```python
from build123d import *

# Parameters (mm, degrees)
SKETCH1_R               = 2.5
BOSS_EXTRUDE1_DEPTH     = 5
SKETCH2_R               = 2.51348819
BOSS_EXTRUDE2_DEPTH     = 1
BOSS_EXTRUDE3_DEPTH     = 3
CUT_EXTRUDE1_DEPTH      = 28.128538457
CUT_EXTRUDE1_DEPTH_BACK = 28.128538457
SKETCH5_R               = 0.5
CUT_EXTRUDE2_START      = -10
SKETCH6_R               = 1.5
CUT_EXTRUDE2_DEPTH      = 10


with BuildPart() as part:
    # Sketch1 → Boss-Extrude1 (new body)
    with BuildSketch(Plane(origin=(0, 0, -3.289858219), x_dir=(-1, 0, 0), z_dir=(0, 0, -1))):
        with BuildLine():
            Line((2.125597577, 8.274515134), (2.125597577, 18.874515134))
            ThreePointArc((2.125597577, 18.874515134), (5.125597577, 21.874515134), (8.125597577, 18.874515134))
            Line((8.125597577, 18.874515134), (8.125597577, 8.274515134))
            ThreePointArc((8.125597577, 8.274515134), (5.125597577, 5.274515134), (2.125597577, 8.274515134))
        make_face()
        with Locations((5.125597577, 18.874515134)):
            Circle(SKETCH1_R, mode=Mode.SUBTRACT)
        with Locations((5.125597577, 8.274515134)):
            Circle(SKETCH1_R, mode=Mode.SUBTRACT)
    extrude(amount=BOSS_EXTRUDE1_DEPTH)

    # Sketch2 → Boss-Extrude2 (add)
    with BuildSketch(Plane(origin=(0, 0, -3.289858219), x_dir=(-1, 0, 0), z_dir=(0, 0, -1))):
        with Locations((5.139085766, 8.274515134)):
            Circle(SKETCH2_R)
        with Locations((5.139085766, 18.874515134)):
            Circle(SKETCH2_R)
    extrude(amount=BOSS_EXTRUDE2_DEPTH)

    # Sketch4 → Boss-Extrude3 (add)
    with BuildSketch(Plane(origin=(0, 0, -3.289858219), x_dir=(-1, 0, 0), z_dir=(0, 0, -1))):
        with BuildLine():
            Line((-9.960914234, 18.874515134), (-10.460914234, 18.874515134))
            Line((-10.460914234, 18.874515134), (-10.460914234, 8.274515134))
            Line((-10.460914234, 8.274515134), (-9.960914234, 8.274515134))
            ThreePointArc((-9.960914234, 8.274515134), (-8.460914234, 9.774515134), (-6.960914234, 8.274515134))
            Line((-6.960914234, 8.274515134), (5.139085766, 8.274515134))
            Line((5.139085766, 8.274515134), (12.039085766, 8.274515134))
            ThreePointArc((12.039085766, 8.274515134), (13.539085766, 9.774515134), (15.039085766, 8.274515134))
            Line((15.039085766, 8.274515134), (15.539085766, 8.274515134))
            Line((15.539085766, 8.274515134), (15.539085766, 18.874515134))
            Line((15.539085766, 18.874515134), (15.039085766, 18.874515134))
            ThreePointArc((15.039085766, 18.874515134), (13.539085766, 17.374515134), (12.039085766, 18.874515134))
            Line((12.039085766, 18.874515134), (5.139085766, 18.874515134))
            Line((5.139085766, 18.874515134), (-6.960914234, 18.874515134))
            ThreePointArc((-6.960914234, 18.874515134), (-8.460914234, 17.374515134), (-9.960914234, 18.874515134))
        make_face()
        with BuildLine():
            Line((15.539085766, 21.874515134), (5.125597577, 21.874515134))
            Line((5.125597577, 21.874515134), (-10.460914234, 21.874515134))
            Line((-10.460914234, 21.874515134), (-10.460914234, 18.874515134))
            Line((-10.460914234, 18.874515134), (-9.960914234, 18.874515134))
            ThreePointArc((-9.960914234, 18.874515134), (-8.460914234, 20.374515134), (-6.960914234, 18.874515134))
            Line((-6.960914234, 18.874515134), (5.139085766, 18.874515134))
            Line((5.139085766, 18.874515134), (12.039085766, 18.874515134))
            ThreePointArc((12.039085766, 18.874515134), (13.539085766, 20.374515134), (15.039085766, 18.874515134))
            Line((15.039085766, 18.874515134), (15.539085766, 18.874515134))
            Line((15.539085766, 18.874515134), (15.539085766, 21.874515134))
        make_face()
        with BuildLine():
            Line((-9.960914234, 8.274515134), (-10.460914234, 8.274515134))
            Line((-10.460914234, 8.274515134), (-10.460914234, 5.274515134))
            Line((-10.460914234, 5.274515134), (5.125597577, 5.274515134))
            Line((5.125597577, 5.274515134), (15.539085766, 5.274515134))
            Line((15.539085766, 5.274515134), (15.539085766, 8.274515134))
            Line((15.539085766, 8.274515134), (15.039085766, 8.274515134))
            ThreePointArc((15.039085766, 8.274515134), (13.539085766, 6.774515134), (12.039085766, 8.274515134))
            Line((12.039085766, 8.274515134), (5.139085766, 8.274515134))
            Line((5.139085766, 8.274515134), (-6.960914234, 8.274515134))
            ThreePointArc((-6.960914234, 8.274515134), (-8.460914234, 6.774515134), (-9.960914234, 8.274515134))
        make_face()
    extrude(amount=BOSS_EXTRUDE3_DEPTH)

    # Sketch5 → Cut-Extrude1 (cut, two sides: drawn at the far end of the back side and taken through both)
    with BuildSketch(Plane(origin=(0, 0, -4.289858219), x_dir=(-1, 0, 0), z_dir=(0, 0, -1)).offset(-CUT_EXTRUDE1_DEPTH_BACK)):
        with Locations((5.139085766, 20.144515134)):
            Circle(SKETCH5_R)
        with Locations((5.139085766, 17.604515134)):
            Circle(SKETCH5_R)
        with Locations((3.869085766, 8.274515134)):
            Circle(SKETCH5_R)
        with Locations((6.409085766, 8.274515134)):
            Circle(SKETCH5_R)
    extrude(amount=CUT_EXTRUDE1_DEPTH + CUT_EXTRUDE1_DEPTH_BACK, mode=Mode.SUBTRACT)

    # Sketch6 → Cut-Extrude2 (cut)
    with BuildSketch(Plane(origin=(0, 0, -6.289858219), x_dir=(-1, 0, 0), z_dir=(0, 0, -1)).offset(CUT_EXTRUDE2_START)):
        with BuildLine():
            Line((-10.460914234, 5.274515134), (5.125597577, 5.274515134))
            ThreePointArc((5.125597577, 5.274515134), (3.004277233, 6.15319479), (2.125597577, 8.274515134))
            Line((2.125597577, 8.274515134), (2.125597577, 18.874515134))
            ThreePointArc((2.125597577, 18.874515134), (3.004277233, 20.995835477), (5.125597577, 21.874515134))
            Line((5.125597577, 21.874515134), (-10.460914234, 21.874515134))
            Line((-10.460914234, 21.874515134), (-10.460914234, 5.274515134))
        make_face()
        with Locations((-8.460914234, 18.874515134)):
            Circle(SKETCH6_R, mode=Mode.SUBTRACT)
        with Locations((-8.460914234, 8.274515134)):
            Circle(SKETCH6_R, mode=Mode.SUBTRACT)
    extrude(amount=CUT_EXTRUDE2_DEPTH, mode=Mode.SUBTRACT)


solid = part.part
```
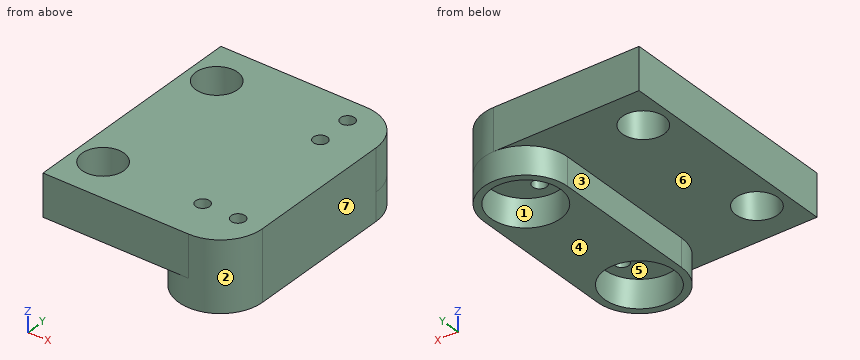
Verification items for the finished model (mm, model axes). Face numbers are marked on the shaded views. A direction names the side the tool comes from. Give positions to 0.01 mm unless a question says otherwise; leave off trailing zeros. Write each loop counter-clockwise with the first axis right and the second up, starting at its lowest first coordinate (ties: lowest second). Pieces come first, ordered by that corner, then holes. Notation, with made-up numbers: (-11, 38) - (32, 38) arc R16 cw to (32, 51) - close; hole circle Ø11 at (-38, 13). An arc over 180 degrees is marked (long way). Put each result on its own line as item: value.
Q1. Depth check by flat-ended pin: P1, Ø2.5, axis at x = -6, y = 7.5, coming from the -Z side; P2, Ø1.8, axis at x = -13.54, y = 18.87, coming from the +Z side; P3, Ø0.6, axis at y = 15.5, z = -7.5, coming from the -X side. Enter the tip coordinate at first touch or a pass-through.
Result:
P1: z = -6.29
P2: through
P3: x = -8.13
Q2. Section check C-C on z = -6.65. Record the cut outline in (x, y).
Result:
outline: (-8.13, 8.27) arc R3 ccw to (-2.13, 8.27) - (-2.13, 18.87) arc R3 ccw to (-8.13, 18.87) - close; hole circle Ø5 at (-5.13, 8.27); hole circle Ø5 at (-5.13, 18.87)
Q3. Section check B-B on x = -14.5. Record the cut outline in (y, z), and give its area (3 significant figures).
Result:
outline: (5.27, -6.29) - (7.12, -6.29) - (7.12, -3.29) - (5.27, -3.29) - close; (9.43, -6.29) - (17.72, -6.29) - (17.72, -3.29) - (9.43, -3.29) - close; (20.03, -6.29) - (21.87, -6.29) - (21.87, -3.29) - (20.03, -3.29) - close
area: 36.0 mm2
Q4. Section check D-D on z = -5.25. Record the cut outline in (x, y), and give its area (3 significant figures).
Result:
outline: (-15.54, 5.27) - (-5.13, 5.27) arc R3 ccw to (-2.13, 8.27) - (-2.13, 18.87) arc R3 ccw to (-5.13, 21.87) - (-15.54, 21.87) - close; hole circle Ø3 at (-13.54, 8.27); hole circle Ø3 at (-13.54, 18.87); hole circle Ø1 at (-6.41, 8.27); hole circle Ø1 at (-5.14, 17.6); hole circle Ø1 at (-5.14, 20.14); hole circle Ø1 at (-3.87, 8.27)
area: 202 mm2
Q5. Set-up check for the marked faces 1, 2, 3 and 4: record each of +Z, -Z, +X, -X, +Y, -Y from which the full face is reachable in a straight line by a thin tool's end or side.
Result:
face 1: -Z
face 2: -Z, -Y
face 3: -Z, -X, +Y, -Y
face 4: -Z, +X, -X, +Y, -Y
Q6. Mould release check, pull along X, two halves, no side actions. Record for the marked faces 5, 6 and 7: released by +X, released by -X, zero draft, split by the parting line, or undercut.
Result:
face 5: undercut
face 6: zero draft
face 7: released by +X
Q7. Section check A-A on y = 7.25. Record the cut outline in (x, z), and give its area (3 significant figures).
Result:
outline: (-15.54, -6.29) - (-14.63, -6.29) - (-14.63, -3.29) - (-15.54, -3.29) - close; (-12.44, -6.29) - (-7.95, -6.29) - (-7.95, -8.29) - (-7.41, -8.29) - (-7.41, -6.29) - (-2.85, -6.29) - (-2.85, -8.29) - (-2.31, -8.29) - (-2.31, -3.29) - (-12.44, -3.29) - close
area: 35.3 mm2
Q8. Scan lines: probe 1 along Y at (x, z) = (-3.25, -7.9); probe 2 along X at (y, z) = (8, -4.8); probe 3 along Y at (x, z) = (-5.5, -5.2). Record each from-to range of solid material in increasing order. Write a range as from..to.
Result:
probe 1: 5.93..6.62, 9.93..17.22, 20.53..21.22
probe 2: -15.54..-15.01, -12.06..-6.83, -5.99..-4.29, -3.45..-2.14
probe 3: 5.27..17.26, 17.95..19.8, 20.49..21.87
